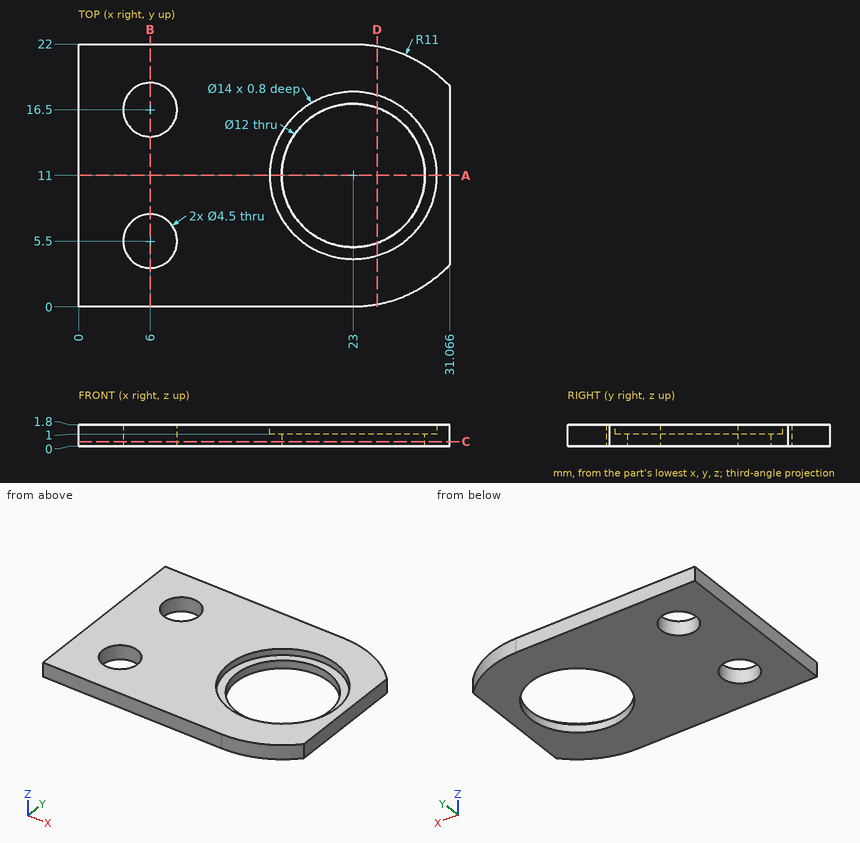
For this review, use the dimensioned drawing (mm, ordinates from the lowest corner) and the shaded views. Coordinates: 2 decimals unless noted, no trailing zeros. Write each loop counter-clockwise with the first axis right and the second up, starting at its lowest first coordinate (ties: lowest second). Pieces come first, ordered by that corner, then holes. Notation, with made-up numbers: (53.5, 64) - (88.5, 64) arc R10 ccw to (88.5, 79) - close; hole circle Ø11 at (-33.75, -9.5). An arc over 180 degrees is marked (long way). Answer in a Markdown table with one row per item. Add a question column.
Q1. Consider section B-B on x = 6. Give the boundary of the cut face in (y, z), then the cut area to 3 significant figures.
Q2. Consider section A-A on y = 11. Give the boundary of the cut face in (x, z).
Q3. Consider section C-C on z = 0.4. Give the boundary of the cut face in (x, y).
Q4. Consider section D-D on x = 25. Give the boundary of the cut face in (y, z).
Q5. To check wall thickness, follow line 1 along Y through (x, z) = (6, 0.5); line 2 along Y through (x, z) = (23, 0.75); line 3 along X through (y, z) = (7.5, 0.25) (1 decimal). State the ranges of each line that lie inside material, in increasing order. Write a range as from..to.
Answers below:
| question | item | result |
|---|---|---|
| 1 | outline | (0, 0) - (3.25, 0) - (3.25, 1.8) - (0, 1.8) - close; (7.75, 0) - (14.25, 0) - (14.25, 1.8) - (7.75, 1.8) - close; (18.75, 0) - (22, 0) - (22, 1.8) - (18.75, 1.8) - close |
| 1 | area | 23.4 mm² |
| 2 | outline | (0, 0) - (17, 0) - (17, 1) - (16, 1) - (16, 1.8) - (0, 1.8) - close; (29, 0) - (31.07, 0) - (31.07, 1.8) - (30, 1.8) - (30, 1) - (29, 1) - close |
| 3 | outline | (0, 0) - (23, 0) arc R11 ccw to (31.07, 3.52) - (31.07, 18.48) arc R11 ccw to (23, 22) - (0, 22) - close; hole circle Ø4.5 at (6, 5.5); hole circle Ø4.5 at (6, 16.5); hole circle Ø12 at (23, 11) |
| 4 | outline | (0.18, 0) - (5.34, 0) - (5.34, 1) - (4.29, 1) - (4.29, 1.8) - (0.18, 1.8) - close; (16.66, 0) - (21.82, 0) - (21.82, 1.8) - (17.71, 1.8) - (17.71, 1) - (16.66, 1) - close |
| 5 | line 1 | 0..3.25, 7.75..14.25, 18.75..22 |
| 5 | line 2 | 0..5, 17..22 |
| 5 | line 3 | 0..5, 7..18.1, 27.9..31.1 |
